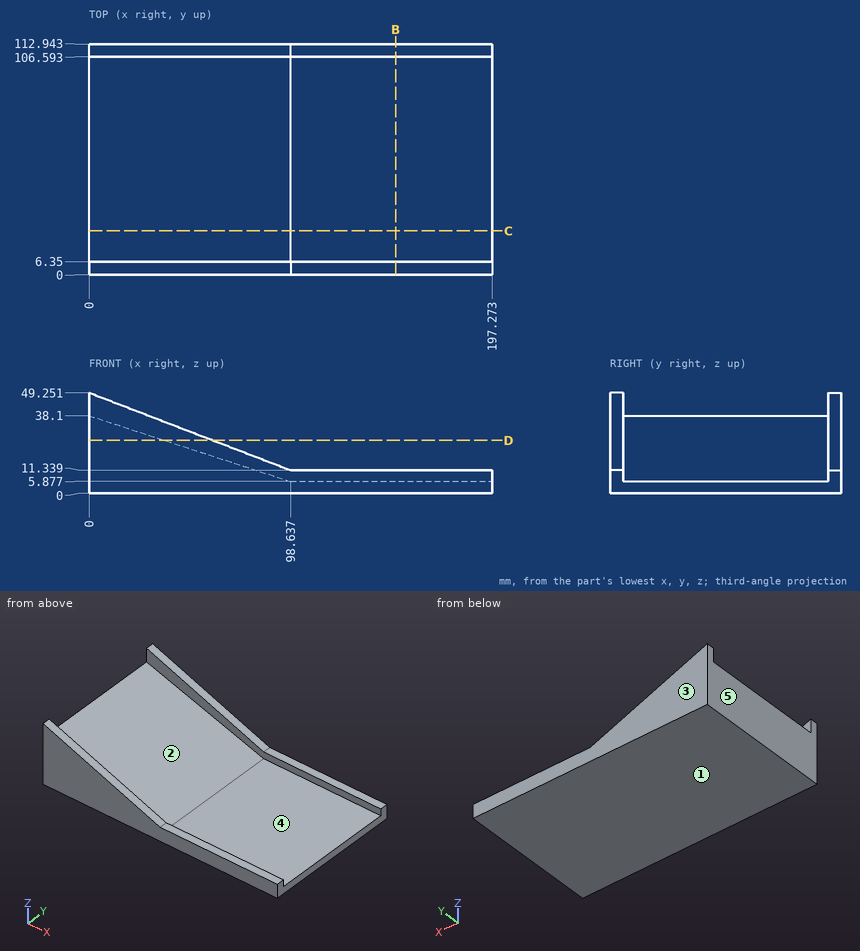
Source: three-view drawing plus pictorial views. Frame: mm from the lowest corner of the part. A direction names the side the tool comes from. Give positions to 0.01 mm unless a question says otherwise; leave off trailing zeros. Order: outer loops, then holes, each group sorted by start corner. A loop starts at its lowest first (then second) coordinate and runs counter-clockwise, first axis right, second up. Notation, with made-up numbers: M 66,-37 L 72,-37 A14 cw 72,-23 Z; hole C 80.5,63.25 d4. An arc over 180 degrees is marked long. One line per question, with ' | ' between items.
1) Ray query, L1, parallel to Y at x = 11.5, z = 44; L2, parallel to Z at x = 104, y = 29.5; L3, parallel to Z at x = 66.5, y = 106.5 (1 decimal). Return the intervals inside material, ascending.
Filled in:
L1: y = 0 to 6.35, 106.59 to 112.94 | L2: z = 0 to 5.88 | L3: z = 0 to 16.4
2) Section B-B on x = 150. Output: boundary loops of the cut face in (y, z), and give its area (3 significant figures).
Filled in:
outline: M 0,0 L 112.94,0 L 112.94,11.34 L 106.59,11.34 L 106.59,5.88 L 6.35,5.88 L 6.35,11.34 L 0,11.34 Z | area: 733 mm2
3) Section C-C on y = 21.5. Output: boundary loops of the cut face in (x, z), and give its area (3 significant figures).
Filled in:
outline: M 0,0 L 197.27,0 L 197.27,5.88 L 98.64,5.88 L 0,38.1 Z | area: 2,750 mm2
4) Contact query for flat-ended pins moving along their axis: P1, Ø1.5, axis at x = 98.5, y = 97, coming from the +Z side; P2, Ø10, axis at y = 87, z = 9.5, coming from the +X side; P3, Ø6, axis at x = 63.5, y = 20, coming from the +Z side (1 decimal); P4, Ø7, axis at x = 126, y = 4, coming from the +Z side. Output: stop coordinate, or through.
Filled in:
P1: stops at z = 6.17 | P2: stops at x = 197.27 | P3: stops at z = 18.3 | P4: stops at z = 11.34
5) Access query for the marked faces 1 and 2. Directions: +Z, -Z, +X, -X, +Y, -Y. A direction counts if a zero-diameter tool reaches every point of the face in a straight line with its end or side. Return the directions, or none.
Filled in:
face 1: -Z, +X, -X, +Y, -Y | face 2: +Z, +X
6) Draft query along Y for the marked faces 3, 4 and 5. Return one class per face: pulls with the +Y half, pulls with the -Y half, needs draft (parallel to the pull), parting line crosses it, or undercut.
Filled in:
face 3: pulls with the +Y half | face 4: undercut | face 5: needs draft
7) Section D-D on z = 26. Output: boundary loops of the cut face in (x, y), and give its area (3 significant figures).
Filled in:
outline: M 0,0 L 60.49,0 L 60.49,6.35 L 37.04,6.35 L 37.04,106.59 L 60.49,106.59 L 60.49,112.94 L 0,112.94 Z | area: 4,480 mm2
